Verification items for the finished model (mm, model axes). A direction names the side the tool comes from. Round coordinates to 2 decimals unless told otherwise and drop trailing zeros. Order: outer loops, then holes, each group sorted by start corner. A loop starts at its lowest first (then second) coordinate and runs counter-clockwise, first axis right, second up. Notation, with made-up numbers: (-30, 6) -> (8, 6) arc R13 cw to (8, 23) -> close; hole circle Ø6 at (72.5, 2.5). An arc over 180 degrees is marked (long way). Return JSON: item names as keys, results as strings. Group by question number.
1) Section check D-D on z = 4.5. Enter the section's corners in (x, y).
2) Draft check along X on faces 1 (the flat face through (8, -8, 2)), 2 (the cylindrical face through (10.85, 6.03, 0.99)), 3 (the cylindrical face through (8.767, -16.856, 0.789)). Enter one of: pulls with the +X half, pulls with the -X half, needs draft (parallel to the pull), parting line crosses it, or undercut.
3) Section check C-C on z = 1. Enter the section's corners in (x, y), plus the area to 3 significant figures.
4) Scan lines: L1, parallel to Y at x = 0, z = 4.8; L2, parallel to Y at x = -7.5, z = 0.5; L3, parallel to Z at x = -4.5, y = -11. Record each from-to range of solid material in increasing order.
5) Section check B-B on x = 0. Enter the section's corners in (y, z), plus the area to 3 significant figures.
6) Tool access check on faces 4 (the flat face through (8, 0, 0)), 5 (the cylindrical face through (-7.37, 6.76, 4.27)). Record the directions out of +Z, -Z, +X, -X, +Y, -Y that give a thin tool (end or side, any length) a straight path to the whole face; none if there is none.
7) Section check A-A on y = 0. Enter the section's corners in (x, z).
8) Depth check by flat-ended pin: pin 1 (2 mm diameter, centred on y = 6, z = 3.5, fed in from +X); pin 2 (4 mm diameter, centred on x = 12.12, y = 7, fed in from +Z); pin 3 (2 mm diameter, centred on y = 13, z = 2, fed in from -X); pin 4 (3 mm diameter, centred on x = -7.5, y = 12.99, fed in from +Z). Enter the tip coordinate at first touch or a pass-through.
```python
from build123d import *

# Parameters (mm, degrees)
SKETCH_1_R      = 19
SKETCH_1_R_2    = 7
SKETCH_1_R_3    = 1.6000000000000003
SKETCH_1_R_4    = 1.6
SKETCH_1_R_5    = 1.5999999999999983
SKETCH_1_R_6    = 1.600000000000001
SKETCH_1_R_7    = 1.6000000000000025
SKETCH_1_R_8    = 1.6000000000000008
EXTRUDE_1_DEPTH = 2
EXTRUDE_2_DEPTH = 7
CHAMFER_1_SIZE  = 0.4


with BuildPart() as part:
    # Sketch 1 → Extrude 1 (new body)
    with BuildSketch(Plane.XY):
        Circle(SKETCH_1_R)
        Circle(SKETCH_1_R_2, mode=Mode.SUBTRACT)
        with Locations((1.71e-15, -14)):
            Circle(SKETCH_1_R_3, mode=Mode.SUBTRACT)
        with Locations((-7.500000000000012, -12.99038105676657)):
            Circle(SKETCH_1_R_4, mode=Mode.SUBTRACT)
        with Locations((-7.499999999999923, 12.990381056766621)):
            Circle(SKETCH_1_R_5, mode=Mode.SUBTRACT)
        with Locations((-12.124355652982107, 7.000000000000055)):
            Circle(SKETCH_1_R_6, mode=Mode.SUBTRACT)
        with Locations((14.999999999999998, -1.5526e-13)):
            Circle(SKETCH_1_R_7, mode=Mode.SUBTRACT)
        with Locations((12.124355652982207, 6.99999999999989)):
            Circle(SKETCH_1_R_8, mode=Mode.SUBTRACT)
    extrude(amount=EXTRUDE_1_DEPTH)

    # Sketch 1_3 → Extrude 2 (add)
    with BuildSketch(Plane.XY):
        with BuildLine():
            Line((-4.999999999999949, 8.660254037844416), (-3.4999999999999645, 6.062177826491091))
            ThreePointArc((-3.499999999999931, 6.0621778264911095), (3.500000000000034, 6.062177826491051), (7, 0))
            Line((7, -7.245e-14), (10, -1.0351e-13))
            ThreePointArc((10, 0), (4.999999999999885, 8.660254037844453), (-5.000000000000229, 8.660254037844254))
        make_face()
        with BuildLine():
            Line((-5.000000000000008, -8.660254037844378), (-3.5000000000000053, -6.062177826491065))
            ThreePointArc((-3.4999999999999707, -6.062177826491087), (-7, 2.262e-14), (-3.499999999999931, 6.0621778264911095))
            Line((-3.4999999999999645, 6.062177826491091), (-4.999999999999949, 8.660254037844416))
            ThreePointArc((-5.000000000000229, 8.660254037844254), (-10, 3.675e-14), (-5.000000000000289, -8.660254037844219))
        make_face()
        with BuildLine():
            ThreePointArc((7, -1.71e-15), (3.500000000000017, -6.062177826491061), (-3.4999999999999707, -6.062177826491087))
            Line((-3.5000000000000053, -6.062177826491065), (-5.000000000000008, -8.660254037844378))
            ThreePointArc((-5.000000000000289, -8.660254037844219), (4.999999999999854, -8.66025403784447), (10, -2.45e-15))
            Line((10, -1.0351e-13), (7, -7.245e-14))
        make_face()
    extrude(amount=EXTRUDE_2_DEPTH)

    # Chamfer 1
    chamfer_1_edges = [part.edges().sort_by_distance(p)[0] for p in [
        (-7, 3.708e-14, 7),
        (5.000000000000295, 8.660254037844211, 7),
        (-19, 2.33e-15, 2),
    ]]
    chamfer(chamfer_1_edges, length=CHAMFER_1_SIZE)


solid = part.part
```
Check result:
{
 "1": {"outline": "circle Ø20 at (0, 0); hole circle Ø14 at (0, 0)"},
 "2": {"face 1": "needs draft", "face 2": "undercut", "face 3": "parting line crosses it"},
 "3": {"outline": "circle Ø38 at (0, 0); hole circle Ø3.2 at (-12.12, 7); hole circle Ø3.2 at (-7.5, -12.99); hole circle Ø3.2 at (-7.5, 12.99); hole circle Ø14 at (0, 0); hole circle Ø3.2 at (0, -14); hole circle Ø3.2 at (12.12, 7); hole circle Ø3.2 at (15, 0)", "area": "932 mm^2"},
 "4": {"L1": "-10 to -7, 7 to 10", "L2": "-17.46 to -14.59, -11.39 to 11.39, 14.59 to 17.46", "L3": "0 to 2"},
 "5": {"outline": "(-19, 0) -> (-15.6, 0) -> (-15.6, 2) -> (-18.6, 2) -> (-19, 1.6) -> close; (-12.4, 0) -> (-7, 0) -> (-7, 6.6) -> (-7.4, 7) -> (-9.6, 7) -> (-10, 6.6) -> (-10, 2) -> (-12.4, 2) -> close; (7, 0) -> (19, 0) -> (19, 1.6) -> (18.6, 2) -> (10, 2) -> (10, 6.6) -> (9.6, 7) -> (7.4, 7) -> (7, 6.6) -> close", "area": "71.1 mm^2"},
 "6": {"face 4": "-Z, +X, -X, +Y, -Y", "face 5": "+Z"},
 "7": {"outline": "(-19, 0) -> (-7, 0) -> (-7, 6.6) -> (-7.4, 7) -> (-9.6, 7) -> (-10, 6.6) -> (-10, 2) -> (-18.6, 2) -> (-19, 1.6) -> close; (7, 0) -> (13.4, 0) -> (13.4, 2) -> (10, 2) -> (10, 6.6) -> (9.6, 7) -> (7.4, 7) -> (7, 6.6) -> close; (16.6, 0) -> (19, 0) -> (19, 1.6) -> (18.6, 2) -> (16.6, 2) -> close"},
 "8": {"pin 1": "x = 8.66", "pin 2": "z = 2", "pin 3": "x = -14.66", "pin 4": "through"}
}
